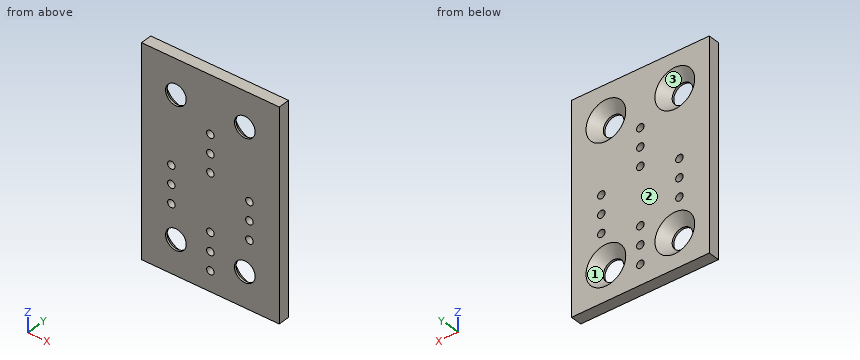
from build123d import *

# Parameters (mm, degrees)
SKETCH2_W                                    = 60
SKETCH2_H                                    = 90
SKETCH2_R                                    = 1.625
BOSS_EXTRUDE1_DEPTH                          = 5
SKETCH3_R                                    = 3.375
CUT_EXTRUDE1_DEPTH                           = 5
CSK_FOR_M8_COUNTERSUNK_FLAT_HEAD_SCR_2_COUNT = 2
CSK_FOR_M8_COUNTERSUNK_FLAT_HEAD_SCR_2_PITCH = 30
CSK_FOR_M8_COUNTERSUNK_FLAT_HEAD_SCR_3_COUNT = 2
CSK_FOR_M8_COUNTERSUNK_FLAT_HEAD_SCR_3_PITCH = 60
CSK_FOR_M8_COUNTERSUNK_FLAT_HEAD_SCR_4_COUNT = 2
CSK_FOR_M8_COUNTERSUNK_FLAT_HEAD_SCR_4_PITCH = 67.082039325


with BuildPart() as part:
    # Sketch2 → Boss-Extrude1 (new body)
    with BuildSketch(Plane(origin=(0, 0, 0), x_dir=(1, 0, 0), z_dir=(0, 1, 0))):
        Rectangle(SKETCH2_W, SKETCH2_H)
        with Locations((0, 20.309068759)):
            Circle(SKETCH2_R, mode=Mode.SUBTRACT)
        with Locations((0, -20.309068759)):
            Circle(SKETCH2_R, mode=Mode.SUBTRACT)
        with Locations((17, 0)):
            Circle(SKETCH2_R, mode=Mode.SUBTRACT)
        with Locations((-17, 0)):
            Circle(SKETCH2_R, mode=Mode.SUBTRACT)
        with Locations((0, 28.309068759)):
            Circle(SKETCH2_R, mode=Mode.SUBTRACT)
        with Locations((17, 8)):
            Circle(SKETCH2_R, mode=Mode.SUBTRACT)
        with Locations((-17, 8)):
            Circle(SKETCH2_R, mode=Mode.SUBTRACT)
        with Locations((0, -12.309068759)):
            Circle(SKETCH2_R, mode=Mode.SUBTRACT)
        with Locations((0, 36.309068759)):
            Circle(SKETCH2_R, mode=Mode.SUBTRACT)
        with Locations((17, 16)):
            Circle(SKETCH2_R, mode=Mode.SUBTRACT)
        with Locations((-17, 16)):
            Circle(SKETCH2_R, mode=Mode.SUBTRACT)
        with Locations((0, -4.309068759)):
            Circle(SKETCH2_R, mode=Mode.SUBTRACT)
    extrude(amount=BOSS_EXTRUDE1_DEPTH)

    # Sketch3 → Cut-Extrude1 (cut)
    with BuildSketch(Plane(origin=(0, 5, 0), x_dir=(1, 0, 0), z_dir=(0, 1, 0))):
        with Locations((-15, 30)):
            Circle(SKETCH3_R)
        with Locations((15, 30)):
            Circle(SKETCH3_R)
        with Locations((15, -30)):
            Circle(SKETCH3_R)
        with Locations((-15, -30)):
            Circle(SKETCH3_R)
    extrude(amount=-CUT_EXTRUDE1_DEPTH, mode=Mode.SUBTRACT)

    # Sketch4 → CSK for M8 Countersunk Flat Head Screw1 (revolve, cut)
    with BuildSketch(Plane(origin=(-15, 5, 30), x_dir=(0, 0, 1), z_dir=(1, 0, 0))):
        Polygon((0, 0), (0, 5), (4.5, 5), (4.5, 4.15), (8.65, 0), align=None)
    csk_for_m8_countersunk_flat_head_screw1 = revolve(axis=Axis((-15, 11.35, 30), (0, -1, 0)), mode=Mode.SUBTRACT)

    # CSK for M8 Countersunk Flat Head Scr 2: CSK for M8 Countersunk Flat Head Screw1 ×2
    with Locations(*[(i * CSK_FOR_M8_COUNTERSUNK_FLAT_HEAD_SCR_2_PITCH, 0, 0) for i in range(1, CSK_FOR_M8_COUNTERSUNK_FLAT_HEAD_SCR_2_COUNT)]):
        add(csk_for_m8_countersunk_flat_head_screw1, mode=Mode.SUBTRACT)

    # CSK for M8 Countersunk Flat Head Scr 3: CSK for M8 Countersunk Flat Head Screw1 ×2
    with Locations(*[(0, 0, -i * CSK_FOR_M8_COUNTERSUNK_FLAT_HEAD_SCR_3_PITCH) for i in range(1, CSK_FOR_M8_COUNTERSUNK_FLAT_HEAD_SCR_3_COUNT)]):
        add(csk_for_m8_countersunk_flat_head_screw1, mode=Mode.SUBTRACT)

    # CSK for M8 Countersunk Flat Head Scr 4: CSK for M8 Countersunk Flat Head Screw1 ×2
    with Locations(*[Vector(0.447213595, 0, -0.894427191) * (i * CSK_FOR_M8_COUNTERSUNK_FLAT_HEAD_SCR_4_PITCH) for i in range(1, CSK_FOR_M8_COUNTERSUNK_FLAT_HEAD_SCR_4_COUNT)]):
        add(csk_for_m8_countersunk_flat_head_screw1, mode=Mode.SUBTRACT)


solid = part.part
Part model, mm, in its own coordinate system. Face numbers are marked on the shaded views. Coordinates: 2 decimals unless noted, no trailing zeros. Loops run counter-clockwise (first coordinate to the right, second up) from the corner with the lowest first, then second, coordinate; pieces in that order, holes last. Notation, with made-up numbers: (38.25, -34.75) - (67.25, -34.75) arc R28 cw to (67.25, -8.75) - close; hole circle Ø6 at (6.25, 62). An arc over 180 degrees is marked (long way). Write each question's results on one line, items separated by ' | '. Start each with the question number.
Q1. Slice it at C-C on y = 1.7. Give the number of separate pieces and of enclosed holes in the cut face, and give its area (3 significant figures).
Q2. Slice it at D-D on z = -8. Give the cut face in (x, y) (3 decimals).
Q3. Two-plate mould, pull along Z, no slides. Class the marked faces 1, 2 and 3: +Z half, -Z half, draft (parallel to the pull), parting line (faces both ways), or undercut.
Q4. Slice it at A-A on z = 30. Give the cut face in (x, y), and give its area (3 significant figures).
Q5. Probe line 1 along X through (y, z) = (0.75, -30); line 2 along X through (y, z) = (4.7, -16) (3 decimals); line 3 along Z through (x, y) = (17, 1.2) (3 decimals). List the from-to ranges inside material, lowest first.
Q6. Slice it at B-B on x = 0. Give the cut face in (y, z).
Answer:
1) separate pieces: 1 | enclosed holes: 16 | area: 4,940 mm2
2) outline: (-30, 0) - (-18.625, 0) - (-18.625, 5) - (-30, 5) - close; (-15.375, 0) - (15.375, 0) - (15.375, 5) - (-15.375, 5) - close; (18.625, 0) - (30, 0) - (30, 5) - (18.625, 5) - close
3) face 1: undercut | face 2: draft | face 3: undercut
4) outline: (-30, 0) - (-19.5, 0) - (-19.5, 0.85) - (-23.65, 5) - (-30, 5) - close; (-10.5, 0) - (10.5, 0) - (10.5, 0.85) - (6.35, 5) - (-6.35, 5) - (-10.5, 0.85) - close; (19.5, 0) - (30, 0) - (30, 5) - (23.65, 5) - (19.5, 0.85) - close | area: 176 mm2
5) line 1: x = -30 to -19.5, -10.5 to 10.5, 19.5 to 30 | line 2: x = -30 to -18.625, -15.375 to 15.375, 18.625 to 30 | line 3: z = -45 to -34.418, -25.582 to -17.625, -14.375 to -9.625, -6.375 to -1.625, 1.625 to 25.582, 34.418 to 45
6) outline: (0, -45) - (5, -45) - (5, -37.93) - (0, -37.93) - close; (0, -34.68) - (5, -34.68) - (5, -29.93) - (0, -29.93) - close; (0, -26.68) - (5, -26.68) - (5, -21.93) - (0, -21.93) - close; (0, -18.68) - (5, -18.68) - (5, 2.68) - (0, 2.68) - close; (0, 5.93) - (5, 5.93) - (5, 10.68) - (0, 10.68) - close; (0, 13.93) - (5, 13.93) - (5, 18.68) - (0, 18.68) - close; (0, 21.93) - (5, 21.93) - (5, 45) - (0, 45) - close
